from build123d import *

# Parameters (mm, degrees)
SKETCH1_W           = 6.25
SKETCH1_H           = 2.5
SKETCH1_W_2         = 9
BOSS_EXTRUDE1_DEPTH = 45


with BuildPart() as part:
    # Sketch1 → Boss-Extrude1 (new body)
    with BuildSketch(Plane.XY):
        Polygon((-3.202898551, 2.789855072), (-3.202898551, 0.289855072), (3.047101449, 0.289855072), (14.797101449, 0.289855072), (14.797101449, 2.789855072), align=None)
        with Locations((-0.077898551, -0.960144928)):
            Rectangle(SKETCH1_W, SKETCH1_H)
        with Locations((1.297101449, -3.460144928)):
            Rectangle(SKETCH1_W_2, SKETCH1_H)
    boss_extrude1 = extrude(amount=BOSS_EXTRUDE1_DEPTH)

    # Mirror1: Boss-Extrude1 across plane
    add(boss_extrude1.mirror(Plane(origin=(14.797101449, 0, 45), x_dir=(0, 0, 1), z_dir=(-1, 0, 0))))

    # Cut-Extrude1 cone 1 section (through the dimple's axis) → Cut-Extrude1 (revolve, cut)
    with BuildSketch(Plane(origin=(14.797101449, 0.289855072, 32.5), x_dir=(0, 0, -1), z_dir=(1, 0, 0))):
        Polygon((0, 0), (1.25, 0), (0, 1.25), align=None)
    revolve(axis=Axis((14.797101449, 0.289855072, 32.5), (0, 1, 0)), mode=Mode.SUBTRACT)

    # Cut-Extrude1 cone 2 section (through the dimple's axis) → Cut-Extrude1 cone 2 (revolve, cut)
    with BuildSketch(Plane(origin=(14.797101449, 0.289855072, 12.5), x_dir=(0, 0, -1), z_dir=(1, 0, 0))):
        Polygon((0, 0), (1.25, 0), (0, 1.25), align=None)
    revolve(axis=Axis((14.797101449, 0.289855072, 12.5), (0, 1, 0)), mode=Mode.SUBTRACT)


solid = part.part
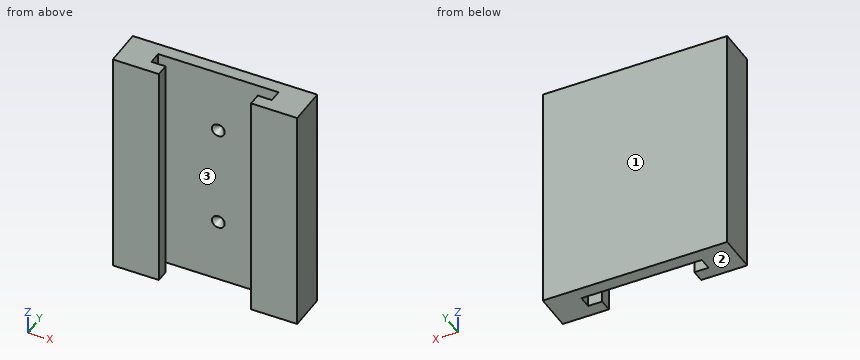
The listing builds one solid part. Answer for the finished solid, in the listing's coordinates (mm). Face numbers are marked on the shaded views. Coordinates: 2 decimals unless noted, no trailing zeros. Loops run counter-clockwise (first coordinate to the right, second up) from the corner with the lowest first, then second, coordinate; pieces in that order, holes last. Notation, with made-up numbers: (2.5, -40) -> (58.5, -40) arc R24 ccw to (58.5, -26) -> close; hole circle Ø6 at (-24, 45). An arc over 180 degrees is marked (long way). Answer in a Markdown table with one row per item. Add a question column.
1. The part is cut by section B-B, the plane x = 25.5. Write down the section's boundary in (y, z), then the cut area to 3 significant figures.
2. Determine the mould class of the marked faces 1, 2 and 3 for opening direction Y: +Y half, -Y half, draft (parallel to the pull), parting line (faces both ways), or undercut.
3. The part is cut by section D-D, the plane x = 8.5. Write down the section's boundary in (y, z), then the cut area to 4 significant figures.
4. Consider line 1 (X direction, y = -1, z = 39); line 2 (X direction, y = -3.5, z = 10.5); line 3 (Y direction, x = 25, z = 35.5). Determine where each line is inside the solid, lowest interval first. Write a range as [from, to].
5. A flat-ended cylindrical pin translates along its axis: P1, Ø2, axis at x = 13.5, z = 24, coming from the -Y side. Find the tip coordinate at first contact, or state that the pin passes through.
6. The part is cut by section A-A, the plane y = -0.25. Write down the section's boundary in (x, z), then the cut area to 4 significant figures.
7. The part is cut by section C-C, the plane z = 26.5. Write down the section's boundary in (x, y), then the cut area to 3 significant figures.
Answer below:
| question | item | result |
|---|---|---|
| 1 | outline | (-4.71, 0) -> (-2.21, 0) -> (-2.21, 45) -> (-4.71, 45) -> close; (0.29, 0) -> (2.79, 0) -> (2.79, 45) -> (0.29, 45) -> close |
| 1 | area | 225 mm2 |
| 2 | face 1 | +Y half |
| 2 | face 2 | draft |
| 2 | face 3 | undercut |
| 3 | outline | (0.29, 0) -> (2.79, 0) -> (2.79, 45) -> (0.29, 45) -> close |
| 3 | area | 112.5 mm2 |
| 4 | line 1 | [-3.2, 3.05], [26.55, 32.8] |
| 4 | line 2 | [-3.2, 5.8], [23.8, 32.8] |
| 4 | line 3 | [-4.71, -2.21], [0.29, 2.79] |
| 5 | P1 | y = 0.29 |
| 6 | outline | (-3.2, 0) -> (3.05, 0) -> (3.05, 45) -> (-3.2, 45) -> close; (26.55, 0) -> (32.8, 0) -> (32.8, 45) -> (26.55, 45) -> close |
| 6 | area | 562.5 mm2 |
| 7 | outline | (-3.2, -4.71) -> (5.8, -4.71) -> (5.8, -2.21) -> (3.05, -2.21) -> (3.05, 0.29) -> (26.55, 0.29) -> (26.55, -2.21) -> (23.8, -2.21) -> (23.8, -4.71) -> (32.8, -4.71) -> (32.8, 2.79) -> (-3.2, 2.79) -> close |
| 7 | area | 166 mm2 |
